Autodesk Inventor part; units mm, degrees
ref_plane "YZ Plane" through (0, 0, 0) normal (1, 0, 0) x (0, 1, 0)
ref_plane "XZ Plane" through (0, 0, 0) normal (0, 1, 0) x (-1, 0, 0)
ref_plane "XY Plane" through (0, 0, 0) normal (0, 0, 1) x (1, 0, 0)
sketch "Sketch1" plane through (0, 0, 0) normal (0, 0, 1) x (1, 0, 0)
  circle A0 centre (0, 0) radius 12.065
  dimension "d0" = 24.13
extrude "Extrusion1" add sketch "Sketch1" along normal blind 24.13
sketch "Sketch2" plane through (0, 0, 24.13) normal (0, 0, 1) x (1, 0, 0)
  circle A0 centre (0, 0) radius 12.065
  circle A1 centre (0, 0) radius 9.525
  dimension "d4" = 19.05
extrude "Extrusion2" add sketch "Sketch2" along normal blind 2.54 contours A1
sketch "Sketch3" plane through (0, 0, 26.67) normal (0, 0, 1) x (1, 0, 0)
  circle A0 centre (0, 0) radius 9.525
  circle A1 centre (0, 0) radius 3.175
  dimension "d8" = 6.35
extrude "Extrusion3" add sketch "Sketch3" along normal blind 1.27 contours A1
sketch "Sketch4" plane through (0, 0, 27.94) normal (0, 0, 1) x (1, 0, 0)
  circle A0 centre (0, 0) radius 3.175
  circle A1 centre (0, 0) radius 0.635
  dimension "d12" = 1.27
extrude "Extrusion4" add sketch "Sketch4" along normal blind 6.35 contours A1
fillet "Fillet1" radius 1.27 2 edges at (-12.065, 0, 24.13) (-9.525, 0, 26.67)
fillet "Fillet2" radius 0.635 1 edges at (-9.525, 0, 24.13)
fillet "Fillet3" radius 0.254 1 edges at (-3.175, 0, 26.67)
properties part number "Motor"
Build history of the part. All positions in model axes, mm. A direction names the side the tool comes from. Round coordinates to 2 decimals unless told otherwise and drop trailing zeros. Write each loop counter-clockwise with the first axis right and the second up, starting at its lowest first coordinate (ties: lowest second). Pieces come first, ordered by that corner, then holes.
1) Pin check, flat tips, straight feed: pin 1 (6 mm diameter, centred on x = 2, y = 7, fed in from +Z); pin 2 (1.5 mm diameter, centred on y = 1, z = 12, fed in from -X); pin 3 (10 mm diameter, centred on x = -1, y = -8, fed in from +Z). Stop position of each tip, or through.
2) Band-saw the part on C-C, the plane z = 5.5. List the corners of the cut face in (x, y) (3 decimals), and give its area (3 significant figures).
3) Drill centre lines: probe 1 along Z at (x, y) = (-9, -6.25); probe 2 along Z at (x, y) = (-1, 3.25); probe 3 along Y at (x, z) = (0.75, 7). Where is each one in solid material? Low to high.
4) Band-saw the part on A-A, the plane x = 0. List the corners of the cut face in (y, z) (3 decimals).
5) 3-axis set-ups, long thin cutter, end or side, ignore diameter. For faces 1 (the flat face through (0, 0, 0)), 2 (the cylindrical face through (-0.08, -0.63, 31.07)): which of +Z, -Z, +X, -X, +Y, -Y reach the whole face in a straight line?
Ans:
1. pin 1: stops at z = 26.67
1. pin 2: stops at x = -12.06
1. pin 3: stops at z = 27.94
2. outline: circle Ø24.13 at (0, 0)
2. area: 457 mm2
3. probe 1: z = 0 to 24.12
3. probe 2: z = 0 to 26.67
3. probe 3: y = -12.04 to 12.04
4. outline: (-12.065, 0) - (12.065, 0) - (12.065, 22.86) arc R1.27 ccw to (10.795, 24.13) - (10.16, 24.13) arc R0.635 cw to (9.525, 24.765) - (9.525, 25.4) arc R1.27 ccw to (8.255, 26.67) - (3.429, 26.67) arc R0.254 cw to (3.175, 26.924) - (3.175, 27.94) - (0.635, 27.94) - (0.635, 34.29) - (-0.635, 34.29) - (-0.635, 27.94) - (-3.175, 27.94) - (-3.175, 26.924) arc R0.254 cw to (-3.429, 26.67) - (-8.255, 26.67) arc R1.27 ccw to (-9.525, 25.4) - (-9.525, 24.765) arc R0.635 cw to (-10.16, 24.13) - (-10.795, 24.13) arc R1.27 ccw to (-12.065, 22.86) - close
5. face 1: -Z, +X, -X, +Y, -Y
5. face 2: +Z
